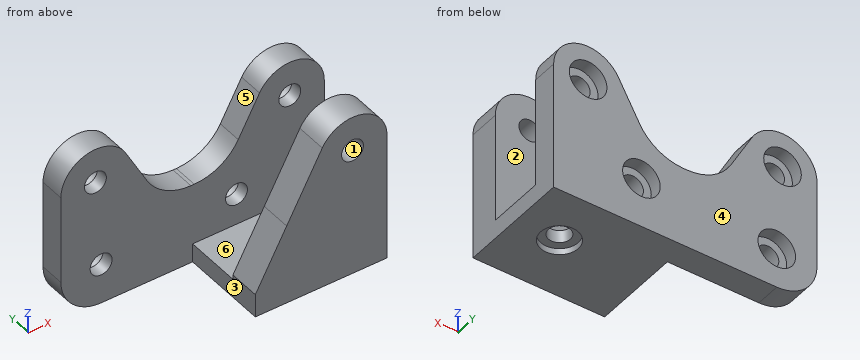
from build123d import *

# Parameters (mm, degrees)
SKETCH1_R           = 1.75
BOSS_EXTRUDE1_DEPTH = 18
SKETCH2_R           = 3
CUT_EXTRUDE1_DEPTH  = 2
CUT_EXTRUDE2_START  = -3
SKETCH4_W           = 42
SKETCH4_H           = 9
CUT_EXTRUDE2_DEPTH  = 35.960505792
CUT_EXTRUDE3_DEPTH  = 14
FILLET1_R           = 8
CUT_EXTRUDE4_DEPTH  = 37.235341864
SKETCH8_R           = 1.75
CUT_EXTRUDE5_DEPTH  = 7
SKETCH9_R           = 1.75
CUT_EXTRUDE6_DEPTH  = 10
SKETCH10_R          = 3
CUT_EXTRUDE7_DEPTH  = 2
SKETCH11_R          = 3
CUT_EXTRUDE8_DEPTH  = 1
FILLET2_R           = 6.41


with BuildPart() as part:
    # Sketch1 → Boss-Extrude1 (new body)
    with BuildSketch(Plane(origin=(0, 0, 0), x_dir=(1, 0, 0), z_dir=(0, 1, 0))):
        with BuildLine():
            Line((-21, 0), (21, 0))
            Line((21, 0), (21, -20.5))
            ThreePointArc((21, -20.5), (16.867011836, -25.827408248), (10.67953504, -23.148229139))
            Line((10.67953504, -23.148229139), (5, -12.81))
            Line((5, -12.81), (-5, -12.81))
            Line((-5, -12.81), (-10.67953504, -23.148229139))
            ThreePointArc((-10.67953504, -23.148229139), (-16.867011836, -25.827408248), (-21, -20.5))
            Line((-21, -20.5), (-21, 0))
        make_face()
        with Locations(Location((15.5, -20.5, 0), (0, 0, 270))):
            Circle(SKETCH1_R, mode=Mode.SUBTRACT)
        with Locations(Location((-15.5, -20.5, 0), (0, 0, 270))):
            Circle(SKETCH1_R, mode=Mode.SUBTRACT)
    extrude(amount=BOSS_EXTRUDE1_DEPTH)

    # Sketch2 → Cut-Extrude1 (cut)
    with BuildSketch(Plane(origin=(0, 18, 0), x_dir=(1, 0, 0), z_dir=(0, 1, 0))):
        with Locations(Location((-15.5, -20.5, 0), (0, 0, 270))):
            Circle(SKETCH2_R)
        with Locations(Location((15.5, -20.5, 0), (0, 0, 270))):
            Circle(SKETCH2_R)
    extrude(amount=-CUT_EXTRUDE1_DEPTH, mode=Mode.SUBTRACT)

    # Sketch4 → Cut-Extrude2 (cut, through all)
    with BuildSketch(Plane(origin=(0, 0, 0), x_dir=(-1, 0, 0), z_dir=(0, 0, -1)).offset(CUT_EXTRUDE2_START)):
        with Locations((0, 9.5)):
            Rectangle(SKETCH4_W, SKETCH4_H)
    extrude(amount=-CUT_EXTRUDE2_DEPTH, mode=Mode.SUBTRACT)

    # Sketch6 → Cut-Extrude3 (cut)
    with BuildSketch(Plane.XZ):
        Polygon((5, 12.81), (-2.037457082, 0), (-21, 0), (-21, 28.272610559), (5, 28.272610559), align=None)
    extrude(amount=-CUT_EXTRUDE3_DEPTH, mode=Mode.SUBTRACT)

    # Fillet1
    fillet1_edges = [part.edges().sort_by_distance(p)[0] for p in [
        (5, 16, 12.81),
        (-5, 16, 12.81),
    ]]
    fillet(fillet1_edges, radius=FILLET1_R)

    # Sketch7 → Cut-Extrude4 (cut, through all)
    with BuildSketch(Plane.XZ.offset(-14)):
        Polygon((0, 0), (0, 4.340639875), (-2.037457082, 0), align=None)
    extrude(amount=CUT_EXTRUDE4_DEPTH, mode=Mode.SUBTRACT)

    # Sketch8 → Cut-Extrude5 (cut)
    with BuildSketch(Plane(origin=(0, 0, 0), x_dir=(-1, 0, 0), z_dir=(0, 0, -1))):
        with Locations((-14, 9.5)):
            Circle(SKETCH8_R)
    extrude(amount=-CUT_EXTRUDE5_DEPTH, mode=Mode.SUBTRACT)

    # Sketch9 → Cut-Extrude6 (cut)
    with BuildSketch(Plane(origin=(0, 18, 0), x_dir=(1, 0, 0), z_dir=(0, 1, 0))):
        with Locations(Location((7, -8, 0), (0, 0, 270))):
            Circle(SKETCH9_R)
        with Locations(Location((-14.59, -6.41, 0), (0, 0, 270))):
            Circle(SKETCH9_R)
    extrude(amount=-CUT_EXTRUDE6_DEPTH, mode=Mode.SUBTRACT)

    # Sketch10 → Cut-Extrude7 (cut)
    with BuildSketch(Plane(origin=(0, 18, 0), x_dir=(1, 0, 0), z_dir=(0, 1, 0))):
        with Locations(Location((7, -8, 0), (0, 0, 270))):
            Circle(SKETCH10_R)
        with Locations(Location((-14.59, -6.41, 0), (0, 0, 270))):
            Circle(SKETCH10_R)
    extrude(amount=-CUT_EXTRUDE7_DEPTH, mode=Mode.SUBTRACT)

    # Sketch11 → Cut-Extrude8 (cut)
    with BuildSketch(Plane(origin=(0, 0, 0), x_dir=(-1, 0, 0), z_dir=(0, 0, -1))):
        with Locations((-14, 9.5)):
            Circle(SKETCH11_R)
    extrude(amount=-CUT_EXTRUDE8_DEPTH, mode=Mode.SUBTRACT)

    # Fillet2
    fillet2_edges = [part.edges().sort_by_distance(p)[0] for p in [
        (-21, 16, 0),
    ]]
    fillet(fillet2_edges, radius=FILLET2_R)


solid = part.part
CAD build for the part. Positions are in the model's coordinates, mm. Face numbers are marked on the shaded views. A direction names the side the tool comes from. Give positions to 0.01 mm unless a question says otherwise; leave off trailing zeros. Loops run counter-clockwise (first coordinate to the right, second up) from the corner with the lowest first, then second, coordinate; pieces in that order, holes last. Notation, with made-up numbers: M 53,32 L 107,32 A13 cw 107,53 Z; hole C 68.25,-21.75 d9. An arc over 180 degrees is marked long. One line per question, with ' | ' between items. Start each with the question number.
1. Probe L1, parallel to Y at x = 14, z = 2; L2, parallel to Y at x = 9.5, z = 9; L3, parallel to X at y = 16.75, z = 6.41. List the from-to ranges inside material, lowest first. Write a range as from..to.
2. Saw through at A-A on x = -15.5. Give the cut face in (y, z), plus the area to 3 significant figures.
3. Two-plate mould, pull along X, no slides. Class the marked faces 1, 2 and 3: pulls with the +X half, pulls with the -X half, needs draft (parallel to the pull), parting line crosses it, or undercut.
4. Saw through at C-C on z = 7.5. Give the cut face in (x, y).
5. Saw through at B-B on y = 2.75. Give the cut face in (x, z), plus the area to 3 significant figures.
6. 3-axis set-ups, long thin cutter, end or side, ignore diameter. For the marked faces 4, 5 and 6: which of +Z, -Z, +X, -X, +Y, -Y reach the whole face in a straight line?
7. Flat gauge pins, fed straight in: pin 1 (2 mm diameter, centred on y = 7.5, z = 16, fed in from +X); pin 2 (5.5 mm diameter, centred on x = -14.59, z = 6.41, fed in from +Y); pin 3 (5.5 mm diameter, centred on x = 14, y = 9.5, fed in from -Z); pin 4 (1.9 mm diameter, centred on y = 8.5, z = 2.5, fed in from -X). Where does each tip first touch, or does it go through?
8. Saw through at D-D on z = 12. Give the cut face in (x, y) (3 decimals).
Result sheet:
1) L1: y = 0..7.75, 11.25..18 | L2: y = 0..5, 14..16 | L3: x = -21..-17.59, -11.59..4.46, 9.54..21
2) outline: M 14,0.06 L 18,0.06 L 18,3.55 L 16,3.55 L 16,4.92 L 14,4.92 Z; M 14,7.9 L 16,7.9 L 16,9.27 L 18,9.27 L 18,17.5 L 16,17.5 L 16,18.75 L 14,18.75 Z; M 14,22.25 L 16,22.25 L 16,23.5 L 18,23.5 L 18,26 L 14,26 Z | area: 67.3 mm^2
3) face 1: undercut | face 2: needs draft | face 3: pulls with the -X half
4) outline: M -21,14 L -15.96,14 L -15.96,16 L -17.38,16 L -17.38,18 L -21,18 Z; M -13.22,14 L 5.32,14 L 5.32,16 L 4.04,16 L 4.04,18 L -11.8,18 L -11.8,16 L -13.22,16 Z; M 2.08,0 L 21,0 L 21,5 L 2.08,5 Z; M 8.68,14 L 21,14 L 21,18 L 9.96,18 L 9.96,16 L 8.68,16 Z
5) outline: M 0,0 L 21,0 L 21,20.5 A5.5 ccw 10.68,23.15 L 0,3.71 Z; hole C 15.5,20.5 d3.5 | area: 392 mm^2
6) face 4: +Z, -Z, +X, -X, +Y | face 5: +Z, +Y, -Y | face 6: +Z, +X, -X
7) pin 1: passes through | pin 2: stops at y = 16 | pin 3: stops at z = 1 | pin 4: stops at x = 0
8) outline: M -21,14 L 21,14 L 21,18 L -21,18 Z; M 4.555,0 L 21,0 L 21,5 L 4.555,5 Z
